Could you check a few things on this drawing? It's one solid part, dimensions in mm from its lowest x, y, z. Give positions to 0.01 mm unless a question says otherwise; leave off trailing zeros. Loops run counter-clockwise (first coordinate to the right, second up) from the corner with the lowest first, then second, coordinate; pieces in that order, holes last. Notation, with made-up numbers: M -29,-5 L 23,-5 A18 ccw 23,18 Z; hole C -13,-9 d10. An arc over 180 degrees is marked long. Return JSON: item names as keys, results as strings. Group by question number.
1. If we section it at B-B (z = 0.7): Write out the boundary of the cut face in (x, y), plus the area to 3 significant figures.
2. If we section it at A-A (x = 51.5): Write out the boundary of the cut face in (y, z).
3. For pin 1 (8 mm diameter, centred on x = 84, y = 95.5, fed in from -Z); pin 2 (1.5 mm diameter, centred on y = 33, z = 2, fed in from -X); pin 3 (1.5 mm diameter, centred on y = 33.5, z = 1.5, fed in from +X), each with a flat end and sliding along its axis, tell me the tip position at first contact or that it passes through.
4. Please list where these lines run through material, in increasing order: line 1 (Y direction, x = 67.5, z = 1.9); line 2 (X direction, y = 141, z = 1); line 3 (X direction, y = 16, z = 0.35).
5. If we section it at C-C (y = 49): Write out the boundary of the cut face in (x, z), plus the area to 3 significant figures.
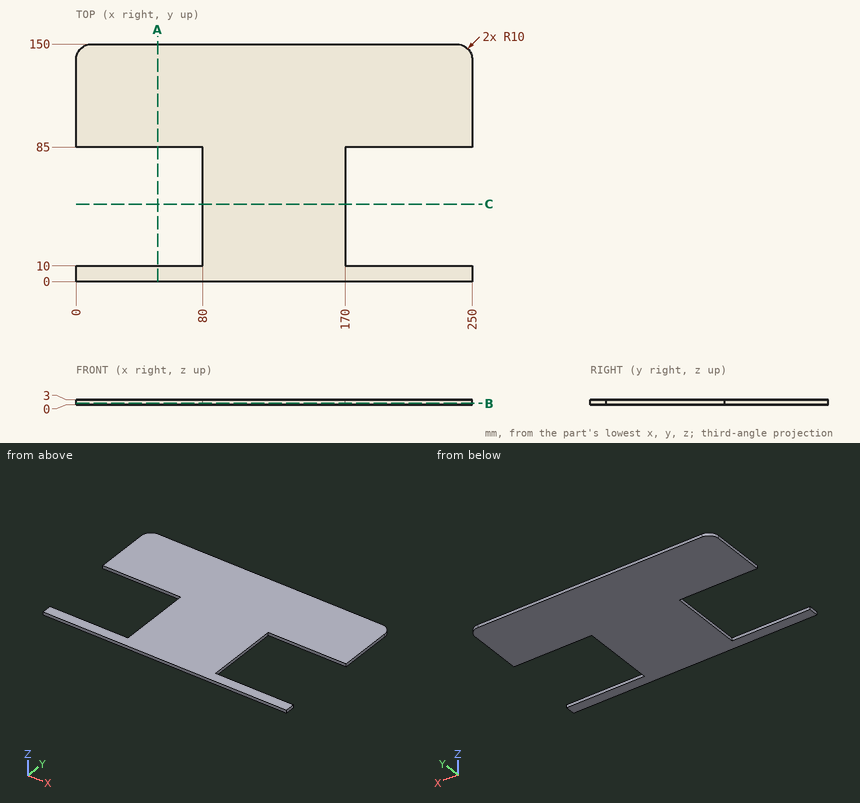
Answer:
{
 "1": {"outline": "M 0,0 L 250,0 L 250,10 L 170,10 L 170,85 L 250,85 L 250,140 A10 ccw 240,150 L 10,150 A10 ccw 0,140 L 0,85 L 80,85 L 80,10 L 0,10 Z", "area": "25,500 mm²"},
 "2": {"outline": "M 0,0 L 10,0 L 10,3 L 0,3 Z; M 85,0 L 150,0 L 150,3 L 85,3 Z"},
 "3": {"pin 1": "stops at z = 0", "pin 2": "stops at x = 80", "pin 3": "stops at x = 170"},
 "4": {"line 1": "y = 0 to 10, 85 to 150", "line 2": "x = 0.05 to 249.95", "line 3": "x = 80 to 170"},
 "5": {"outline": "M 80,0 L 170,0 L 170,3 L 80,3 Z", "area": "270 mm²"}
}
